Autodesk Inventor part; units mm, degrees
ref_plane "YZ Plane" through (0, 0, 0) normal (1, 0, 0) x (0, 1, 0)
ref_plane "XZ Plane" through (0, 0, 0) normal (0, 1, 0) x (-1, 0, 0)
ref_plane "XY Plane" through (0, 0, 0) normal (0, 0, 1) x (1, 0, 0)
sketch "スケッチ1" plane through (0, 0, 0) normal (0, 1, 0) x (-1, 0, 0)
  line L0 (7, 4.5) -> (-7, 4.5)
  line L1 (-7, 4.5) -> (-7, -4.5)
  line L2 (-7, -4.5) -> (7, -4.5)
  line L3 (7, -4.5) -> (7, 4.5)
  line L4 (7, 4.5) -> (-7, -4.5) construction
  line L5 (-7, 4.5) -> (7, -4.5) construction
  point P0 (0, 0)
  dimension "d0" = 14
  dimension "d1" = 9
extrude "押し出し1" add sketch "スケッチ1" along normal blind 8.7
sketch "スケッチ2" plane through (0, 8.7, 0) normal (0, 1, 0) x (1, 0, 0)
  line L0 (7.5, -5.25) -> (-7.5, -5.25)
  line L1 (-7.5, -5.25) -> (-7.5, 5.25)
  line L2 (-7.5, 5.25) -> (7.5, 5.25)
  line L3 (7.5, 5.25) -> (7.5, -5.25)
  line L4 (7.5, -5.25) -> (-7.5, 5.25) construction
  line L5 (-7.5, -5.25) -> (7.5, 5.25) construction
  point P0 (0, 0)
  dimension "d4" = 10.5
  dimension "d5" = 15
extrude "押し出し2" add sketch "スケッチ2" along normal blind 1.3
sketch "スケッチ3" plane through (0, 0, 0) normal (0, -1, 0) x (1, 0, 0)
  line L0 (5.5, 1.95) -> (6, 1.95)
  line L1 (6, 1.95) -> (6, -1.95)
  line L2 (6, -1.95) -> (5.5, -1.95)
  line L3 (5.5, -1.95) -> (5.5, 1.95)
  line L4 (1, 1.95) -> (1.5, 1.95)
  line L5 (1.5, 1.95) -> (1.5, -1.95)
  line L6 (1.5, -1.95) -> (1, -1.95)
  line L7 (1, -1.95) -> (1, 1.95)
  line L8 (7, 4.5) -> (7, -4.5)
  point P0 (0, 0)
  point P1 (1, 0)
  point P2 (6, 0)
  point P3 (7, 0)
  dimension "d10" = 4
  dimension "d11" = 0.5
  dimension "d12" = 3.9
  dimension "d13" = 1
extrude "押し出し3" add sketch "スケッチ3" along normal blind 7
fillet "フィレット1" radius 1 4 edges at (5.75, -7, -1.95) (5.75, -7, 1.95) (1.25, -7, -1.95) (1.25, -7, 1.95)
properties part number "switch"
The model under review builds one solid part; all positions refer to its coordinate system, in mm. A direction names the side the tool comes from. Round coordinates to 2 decimals unless told otherwise and drop trailing zeros. Loops run counter-clockwise (first coordinate to the right, second up) from the corner with the lowest first, then second, coordinate; pieces in that order, holes last. Notation, with made-up numbers: M 22,-8 L 48,-8 A27 ccw 48,8 Z; hole C -13,8 d10. An arc over 180 degrees is marked long. Answer as a JSON object with one key per item and string values.
Item 1: We need section A-A, the plane y = -2.5. State the section outline as (x, z) points.
Check sheet entries:
{"outline": "M 1,-1.95 L 1.5,-1.95 L 1.5,1.95 L 1,1.95 Z; M 5.5,-1.95 L 6,-1.95 L 6,1.95 L 5.5,1.95 Z"}
Item 2: Clearance check with flat-ended pins moving along their axes: P1, Ø0.6, axis at x = 1, y = -3, coming from the -Z side; P2, Ø1.2, axis at y = -4, z = -0.5, coming from the +X side; P3, Ø4, axis at y = 0, z = 0, coming from the +X side. State where each tip first meets the part, or that it passes through.
Check sheet entries:
{"P1": "z = -1.95", "P2": "x = 6", "P3": "x = 7"}
Item 3: Tool access review of faces 1 (the face through (0, 4, 4.5)), 2 (the face through (0, 4, -4.5)), 3 (the face through (1, -3, 0)), 4 (the face through (5.5, -3, 0)), 5 (the face through (6, -3, 0)): name each direction out of +Z, -Z, +X, -X, +Y, -Y from which nothing blocks a thin tool from reaching the whole face with its end or side.
Check sheet entries:
{"face 1": "+Z, +X, -X, -Y", "face 2": "-Z, +X, -X, -Y", "face 3": "+Z, -Z, -X, -Y", "face 4": "+Z, -Z, -Y", "face 5": "+Z, -Z, +X, -Y"}
Item 4: We need section D-D, the plane y = 5.75. State the section outline as (x, z) points, and give its area (3 significant figures).
Check sheet entries:
{"outline": "M -7,-4.5 L 7,-4.5 L 7,4.5 L -7,4.5 Z", "area": "126 mm2"}
Item 5: The part is to be moulded in two halves that separate along X. For faces 6 (the face through (0, 9, -5.25)), 7 (the face through (1.5, -3, 0)), 8 (the face through (-7.5, 9, 0)), say which applies: +X half, -X half, draft (parallel to the pull), parting line (faces both ways), or undercut.
Check sheet entries:
{"face 6": "draft", "face 7": "undercut", "face 8": "-X half"}
Item 6: We need section C-C, the plane x = 4.5. State the section outline as (y, z) points.
Check sheet entries:
{"outline": "M 0,-4.5 L 8.7,-4.5 L 8.7,-5.25 L 10,-5.25 L 10,5.25 L 8.7,5.25 L 8.7,4.5 L 0,4.5 Z"}
Item 7: For line 1 along X through (y, z) = (2.5, 2.25); line 2 along X through (y, z) = (-3.5, 1.25); line 3 along Y through (x, z) = (0, -0.25), list the stretches that pass through material, from the lowest coordinate up.
Check sheet entries:
{"line 1": "-7 to 7", "line 2": "1 to 1.5, 5.5 to 6", "line 3": "0 to 10"}
Item 8: We need section B-B, the plane z = -3.5. State the section outline as (x, y) points.
Check sheet entries:
{"outline": "M -7.5,8.7 L -7,8.7 L -7,0 L 7,0 L 7,8.7 L 7.5,8.7 L 7.5,10 L -7.5,10 Z"}
